Could you check a few things on this model? Use its own coordinates, in mm. Face numbers are marked on the shaded views. Round coordinates to 2 decimals unless told otherwise and drop trailing zeros. Loops run counter-clockwise (first coordinate to the right, second up) from the corner with the lowest first, then second, coordinate; pieces in that order, holes last. Notation, with made-up numbers: M -33,60 L -19,60 A26 cw -19,85 Z; hole C 11,21.5 d5. An arc over 180 degrees is marked long. Return JSON: item names as keys, results as strings. Group by question number.
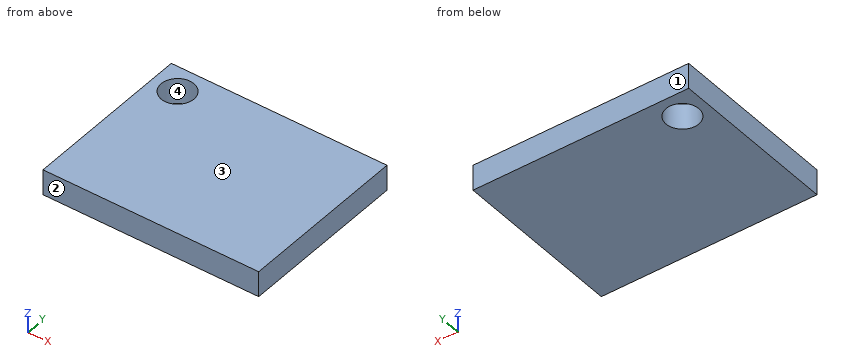
```python
from build123d import *

# Parameters (mm, degrees)
SKETCH1_W             = 21.463
SKETCH1_H             = 16.9164
BOSS_EXTRUDE1_DEPTH   = 2.54
F_4_CLEARANCE_HOLE1_D = 3.2639


with BuildPart() as part:
    # Sketch1 → Boss-Extrude1 (new body)
    with BuildSketch(Plane.XY):
        Rectangle(SKETCH1_W, SKETCH1_H)
    extrude(amount=BOSS_EXTRUDE1_DEPTH)

    # #4 Clearance Hole1 (through all)
    with Locations(Plane.XY.offset(2.54)):
        with Locations((-8.1915, 5.9182)):
            Hole(F_4_CLEARANCE_HOLE1_D / 2)


solid = part.part
```
1. I need wall thicknesses on probe 1 along X at (y, z) = (5.75, 0.65); probe 2 along Y at (x, z) = (-9.25, 1.8); probe 3 along X at (y, z) = (5, 2.3). Which ranges of each line are inside material? Lowest first, please.
2. If we section it at C-C, the plane z = 1.95: Please give me the cut outline in (x, y), then the cut area to 3 significant figures.
3. If we section it at B-B, the plane x = -7.25: Please give me the cut outline in (y, z).
4. If we section it at A-A, the plane y = 7: Please give me the cut outline in (x, z), then the cut area to 3 significant figures.
5. We'd pull the mould along Y, two halves only. Please class the marked faces 1, 2, 3 and 4: +Y half, -Y half, draft (parallel to the pull), parting line (faces both ways), or undercut.
Geometry results:
{
 "1": {"probe 1": "-10.73 to -9.81, -6.57 to 10.73", "probe 2": "-8.46 to 4.68, 7.16 to 8.46", "probe 3": "-10.73 to -9.54, -6.84 to 10.73"},
 "2": {"outline": "M -10.73,-8.46 L 10.73,-8.46 L 10.73,8.46 L -10.73,8.46 Z; hole C -8.19,5.92 d3.26", "area": "355 mm^2"},
 "3": {"outline": "M -8.46,0 L 4.59,0 L 4.59,2.54 L -8.46,2.54 Z; M 7.25,0 L 8.46,0 L 8.46,2.54 L 7.25,2.54 Z"},
 "4": {"outline": "M -10.73,0 L -9.41,0 L -9.41,2.54 L -10.73,2.54 Z; M -6.97,0 L 10.73,0 L 10.73,2.54 L -6.97,2.54 Z", "area": "48.3 mm^2"},
 "5": {"face 1": "+Y half", "face 2": "-Y half", "face 3": "draft", "face 4": "undercut"}
}
